Verification items for this drawing (mm, ordinates from the low corner). A direction names the side the tool comes from. Round coordinates to 2 decimals unless told otherwise and drop trailing zeros. Order: outer loops, then holes, each group sorted by start corner. A loop starts at its lowest first (then second) coordinate and runs counter-clockwise, first axis right, second up. Notation, with made-up numbers: (44.25, -12.5) -> (48.25, -12.5) arc R22 ccw to (48.25, 13.5) -> close; hole circle Ø3 at (57, 89.5). An arc over 180 degrees is marked (long way). Answer in a Markdown table with one row per item.
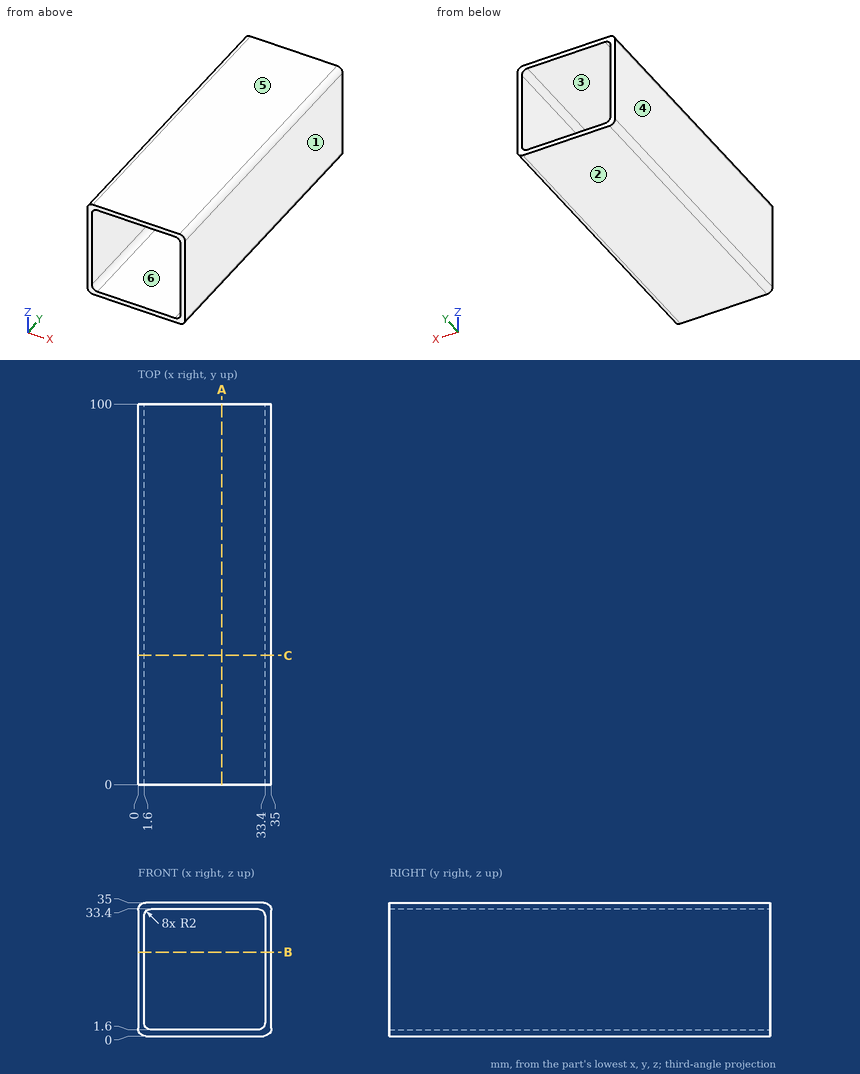
Item 1: Mould release check, pull along X, two halves, no side actions. Record for the marked faces 1, 2, 3 and 4: pulls with the +X half, pulls with the -X half, needs draft (parallel to the pull), parting line crosses it, or undercut.
Result sheet:
| item | result |
|---|---|
| face 1 | pulls with the +X half |
| face 2 | needs draft |
| face 3 | undercut |
| face 4 | pulls with the -X half |
Item 2: Scan lines: line 1 (X direction, y = 64, z = 23); line 2 (X direction, y = 75, z = 32.5). Record each from-to range of solid material in increasing order. Write a range as [from, to].
Result sheet:
| item | result |
|---|---|
| line 1 | x = [0, 1.6], [33.4, 35] |
| line 2 | x = [0, 1.93], [33.07, 35] |
Item 3: Cross-section at C-C (y = 34). Record the boundary of the cut face in (x, z), and give its area (3 significant figures).
Result sheet:
| item | result |
|---|---|
| outline | (0, 2) arc R2 ccw to (2, 0) -> (33, 0) arc R2 ccw to (35, 2) -> (35, 33) arc R2 ccw to (33, 35) -> (2, 35) arc R2 ccw to (0, 33) -> close; hole (1.6, 3.6) arc R2 ccw to (3.6, 1.6) -> (31.4, 1.6) arc R2 ccw to (33.4, 3.6) -> (33.4, 31.4) arc R2 ccw to (31.4, 33.4) -> (3.6, 33.4) arc R2 ccw to (1.6, 31.4) -> close |
| area | 214 mm^2 |
Item 4: Cross-section at A-A (x = 22). Record the boundary of the cut face in (y, z).
Result sheet:
| item | result |
|---|---|
| outline | (0, 0) -> (100, 0) -> (100, 1.6) -> (0, 1.6) -> close; (0, 33.4) -> (100, 33.4) -> (100, 35) -> (0, 35) -> close |
Item 5: Set-up check for the marked faces 5 and 6: record each of +Z, -Z, +X, -X, +Y, -Y from which the full face is reachable in a straight line by a thin tool's end or side.
Result sheet:
| item | result |
|---|---|
| face 5 | +Z, +X, -X, +Y, -Y |
| face 6 | +Y, -Y |
Item 6: Cross-section at B-B (z = 22). Record the boundary of the cut face in (x, y).
Result sheet:
| item | result |
|---|---|
| outline | (0, 0) -> (1.6, 0) -> (1.6, 100) -> (0, 100) -> close; (33.4, 0) -> (35, 0) -> (35, 100) -> (33.4, 100) -> close |
